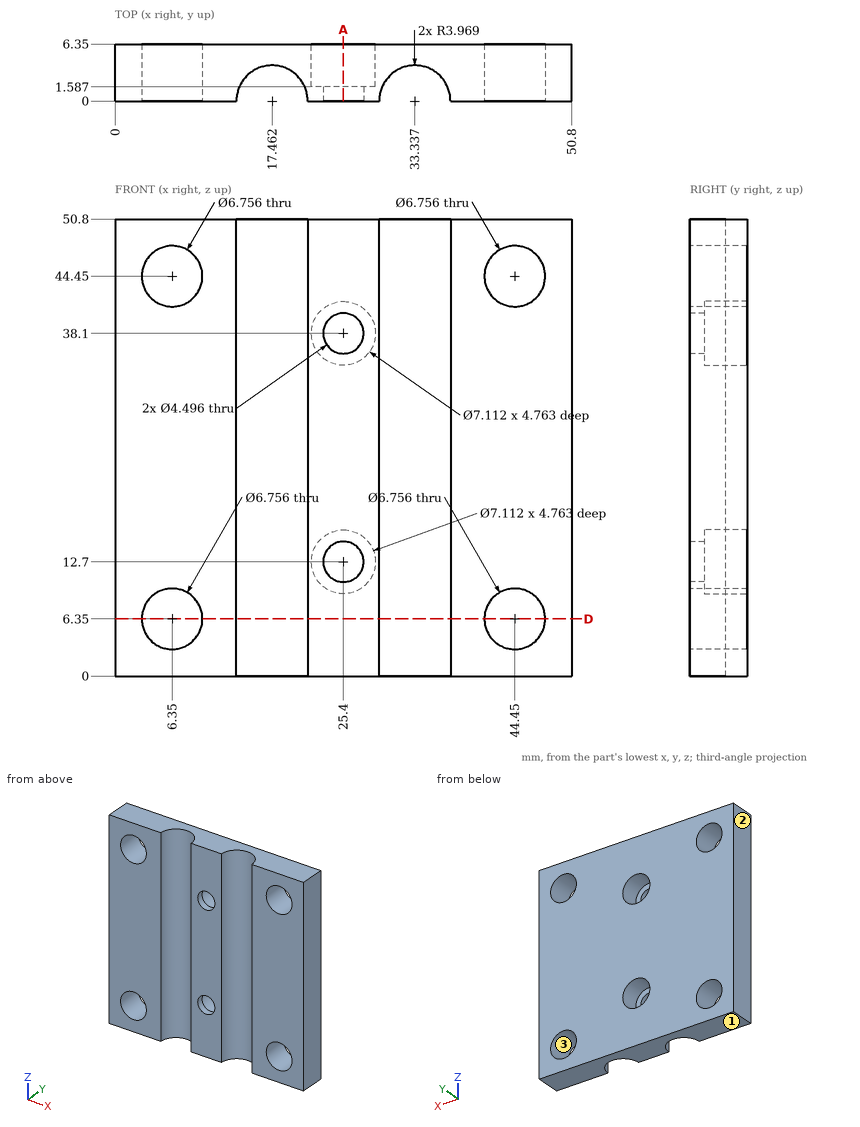
Part print with two shaded views. Sizes in mm from the minimum x, y, z corner. Coordinates: 2 decimals unless noted, no trailing zeros. Write each loop counter-clockwise with the first axis right and the second up, starting at its lowest first coordinate (ties: lowest second). Pieces come first, ordered by that corner, then holes.
(1) Cut at D-D on z = 6.35. List the corners of the cut face in (x, y).
(2) Pin check, flat tip, straight feed: pin 1 Ø6.5 at (x, z) = (25.4, 12.7) entering from +Y. Stop position of the tip, or through.
(3) Mould opens along Z. For the marked faces 1, 2 and 3 say: pulls with the +Z half, pulls with the -Z half, needs draft (parallel to the pull), parting line crosses it, or undercut.
(4) Drill centre lines: line 1 (Z direction, x = 25.4, y = 0.85); line 2 (Z direction, x = 44.45, y = 1.75); line 3 (X direction, y = 1.25, z = 8.5) (1 decimal). Where is each one in solid material? Low to high.
(5) Cut at A-A on x = 25.4. State how many separate pieces and enclosed holes the cut face has.
Working result:
1. outline: (0, 0) - (2.97, 0) - (2.97, 6.35) - (0, 6.35) - close; (9.73, 0) - (13.49, 0) arc R3.97 cw to (21.43, 0) - (29.37, 0) arc R3.97 cw to (37.31, 0) - (41.07, 0) - (41.07, 6.35) - (9.73, 6.35) - close; (47.83, 0) - (50.8, 0) - (50.8, 6.35) - (47.83, 6.35) - close
2. pin 1: stops at y = 1.59
3. face 1: pulls with the -Z half
3. face 2: needs draft
3. face 3: undercut
4. line 1: z = 0 to 10.45, 14.95 to 35.85, 40.35 to 50.8
4. line 2: z = 0 to 2.97, 9.73 to 41.07, 47.83 to 50.8
4. line 3: x = 0 to 3.7, 9 to 13.7, 21.2 to 29.6, 37.1 to 41.8, 47.1 to 50.8
5. separate pieces: 3
5. enclosed holes: 0
